Geometry: final body of the model. Coordinates: model frame, mm. A direction names the side the tool comes from. Coordinates: 2 decimals unless noted, no trailing zeros. Loops run counter-clockwise (first coordinate to the right, second up) from the corner with the lowest first, then second, coordinate; pieces in that order, holes last. Notation, with made-up numbers: (81, 83) - (114, 83) arc R18 cw to (114, 93) - close; hole circle Ø6 at (51.5, 22.5). An arc over 180 degrees is marked (long way). Put each result on its own line as item: value. Start each with the question number.
1) Reachability of faces 5 (the flat face through (32, -6, 57)), 6 (the cylindrical face through (-11.496, -3.451, -13.231)) from +Z, -Z, +X, -X, +Y, -Y: full face, straight path, thin tool, end or side. Return the list, or none.
2) Draft query along X for faces 1 (the cylindrical face through (35.682, -3.451, 8.144)), 2 (the flat face through (25.5, 0, -14.1)), 3 (the cylindrical face through (-9.587, -2.958, 57.133)), 4 (the flat face through (-44.856, -2, 2)). Return one class per face: +X half, -X half, draft (parallel to the pull), parting line (faces both ways), or undercut.
3) Section A-A on y = -2. Count the separate pieces of the cut face and the enclosed holes in it, and give its area (3 significant figures).
4) Section C-C on z = -41. Output: boundary loops of the cut face in (x, y), and give its area (3 significant figures).
5) Material intervals for line 1 along Z through (x, y) = (-40, -2.25); line 2 along X through (y, z) = (-1.25, 43); line 3 along X through (y, z) = (-2.5, -25.5), sorted ascending. Write a range as from..to.
6) Contact query for flat-ended pins moving along their axis: pin 1 Ø1 at (x, z) = (-35, -20) entering from +Y; pin 2 Ø2 at (x, y) = (24.5, -5.5) entering from +Z. Output: stop coordinate, or through.
7) Section B-B on z = -21.5. Output: boundary loops of the cut face in (x, y), and give its area (3 significant figures).
```python
from build123d import *

# Parameters (mm, degrees)
F0_W        = 4
F0_H        = 120
F0_R        = 18
F1_DEPTH    = 7
F2_T1_DEPTH = 135
F2_T3_DEPTH = 99
F3_T        = -1


# Not quite as in the source:
# - a fillet or chamfer that OpenCascade refuses, or shapes differently, is made with other operations: its cross-section is extruded or revolved along the edge and cut away or added


with BuildPart() as f1:
    # F0 (on Front) → F1 (new body)
    with BuildSketch(Plane.XZ):
        with Locations((-42.8557436466, 2.7328292441)):
            Rectangle(F0_W, F0_H)
        Polygon((-0.6441245232, 2.7376232945), (-0.6441245232, 62.7328292441), (-40.8557436466, 62.7328292441), (-40.8557436466, -57.2671707559), (-0.6441245232, -57.2671707559), align=None)
        with Locations((-19.8015584055, -35.636439333)):
            Circle(F0_R, mode=Mode.SUBTRACT)
        with Locations((-19.8015584055, 2.7376232945)):
            Circle(F0_R, mode=Mode.SUBTRACT)
        with Locations((-19.8015584055, 41.1116859221)):
            Circle(F0_R, mode=Mode.SUBTRACT)
        Polygon((39.1442563534, -57.2671707559), (39.1442563534, 62.7328292441), (-0.6441245232, 62.7328292441), (-0.6441245232, 2.7376232945), (-0.6441245232, -57.2671707559), align=None)
        with Locations((18.5133093592, -35.636439333)):
            Circle(F0_R, mode=Mode.SUBTRACT)
        with Locations((18.5133093592, 2.7376232945)):
            Circle(F0_R, mode=Mode.SUBTRACT)
        with Locations((18.5133093592, 41.1116859221)):
            Circle(F0_R, mode=Mode.SUBTRACT)
    extrude(amount=F1_DEPTH)

    # F2: fillet of radius 3 on 4 edges, made by hand

    # F2_s2 → F2_t1 (cut)
    with BuildSketch(Plane.XY.offset(-64.7671707559)):
        with BuildLine():
            ThreePointArc((-44.8557436466, -4), (-43.9770639902, -6.1213203436), (-41.8557436466, -7))
            Line((-41.8557436466, -7), (-44.8557436466, -7))
            Line((-44.8557436466, -7), (-44.8557436466, -4))
        make_face()
        with BuildLine():
            ThreePointArc((39.1442563534, -4), (38.2655766969, -6.1213203436), (36.1442563534, -7))
            Line((36.1442563534, -7), (39.1442563534, -7))
            Line((39.1442563534, -7), (39.1442563534, -4))
        make_face()
    extrude(amount=F2_T1_DEPTH, mode=Mode.SUBTRACT)

    # F2_s4 → F2_t3 (cut)
    with BuildSketch(Plane.YZ.offset(-52.3557436466)):
        with BuildLine():
            ThreePointArc((-4, -57.2671707559), (-6.1213203436, -56.3884910995), (-7, -54.2671707559))
            Line((-7, -54.2671707559), (-7, -57.2671707559))
            Line((-7, -57.2671707559), (-4, -57.2671707559))
        make_face()
        with BuildLine():
            ThreePointArc((-4, 62.7328292441), (-6.1213203436, 61.8541495876), (-7, 59.7328292441))
            Line((-7, 59.7328292441), (-7, 62.7328292441))
            Line((-7, 62.7328292441), (-4, 62.7328292441))
        make_face()
    extrude(amount=F2_T3_DEPTH, mode=Mode.SUBTRACT)

    # F3
    f3_openings = [f1.faces().sort_by_distance(p)[0] for p in [
        (-43.390957, 0, 2.732829),
    ]]
    offset(amount=F3_T, openings=f3_openings)


solid = f1.part
```
Answer block:
1. face 5: +Y
1. face 6: +Y, -Y
2. face 1: undercut
2. face 2: draft
2. face 3: undercut
2. face 4: -X half
3. separate pieces: 7
3. enclosed holes: 7
3. area: 1,100 mm²
4. outline: (-44.86, -4) arc R3 ccw to (-41.86, -7) - (-36.98, -7) - (-36.98, 0) - (-38.03, 0) - (-38.03, -6) - (-41.86, -6) arc R2 cw to (-43.86, -4) - (-43.86, 0) - (-44.86, 0) - close; (-2.62, -7) - (1.33, -7) - (1.33, 0) - (0.29, 0) - (0.29, -6) - (-1.57, -6) - (-1.57, 0) - (-2.62, 0) - close; (35.7, -7) - (36.14, -7) arc R3 ccw to (39.14, -4) - (39.14, 0) - (38.14, 0) - (38.14, -4) arc R2 cw to (36.74, -5.91) - (36.74, 0) - (35.7, 0) - close
4. area: 50.2 mm²
5. line 1: z = -57.27..-56.27, 61.73..62.73
5. line 2: x = -44.86..-43.86, -38.71..-37.7, -1.9..-0.9, -0.39..0.61, 36.41..37.42, 38.14..39.14
5. line 3: x = -44.86..-43.86, -35.87..-34.68, -4.93..-3.73, 2.44..3.64, 33.39..34.58, 38.14..39.14
6. pin 1: stops at y = -6
6. pin 2: stops at z = 62.69
7. outline: (-44.86, -4) arc R3 ccw to (-41.86, -7) - (-30.94, -7) - (-30.94, 0) - (-32.5, 0) - (-32.5, -6) - (-41.86, -6) arc R2 cw to (-43.86, -4) - (-43.86, 0) - (-44.86, 0) - close; (-8.66, -7) - (7.37, -7) - (7.37, 0) - (5.82, 0) - (5.82, -6) - (-7.11, -6) - (-7.11, 0) - (-8.66, 0) - close; (29.66, -7) - (36.14, -7) arc R3 ccw to (39.14, -4) - (39.14, 0) - (38.14, 0) - (38.14, -4) arc R2 cw to (36.14, -6) - (31.21, -6) - (31.21, 0) - (29.66, 0) - close
7. area: 86.5 mm²
